Geometry check sheet. Reference: the model listing, model coordinates, mm. A direction names the side the tool comes from. Round coordinates to 2 decimals unless told otherwise and drop trailing zeros. Write each loop counter-clockwise with the first axis right and the second up, starting at its lowest first coordinate (ties: lowest second). Pieces come first, ordered by that corner, then holes. Notation, with made-up numbers: (74.25, 12) -> (111.25, 12) arc R18 cw to (111.25, 19) -> close; hole circle Ø3 at (61.5, -20). An arc over 180 degrees is marked (long way). Put each result on its own line as item: value. Start each with the question number.
from build123d import *

# Parameters (mm, degrees)
SKETCH041_W             = 20
SKETCH041_H             = 20
PAD030_DEPTH            = 50
PAD030_FACE1_W          = 20
PAD030_FACE1_H          = 50
PAD031_DEPTH            = 100
SKETCH043_W             = 20
SKETCH043_H             = 12
POCKET008_DEPTH         = 100
BODY003_PLACEMENT_ANGLE = 45


with BuildPart() as part:
    # Sketch041 → Pad030 (new body)
    with BuildSketch(Plane.XY):
        with Locations((-89.365005, -120.837763)):
            Rectangle(SKETCH041_W, SKETCH041_H)
    extrude(amount=PAD030_DEPTH)

    # Pad030 Face1 → Pad031 (add)
    with BuildSketch(Plane(origin=(-89.365005, -110.837763, 25), x_dir=(1, 0, 0), z_dir=(0, 1, 0))):
        Rectangle(PAD030_FACE1_W, PAD030_FACE1_H)
    extrude(amount=PAD031_DEPTH)

    # Sketch043 (on Face8 of Pad031) → Pocket008 (cut)
    with BuildSketch(Plane(origin=(0, -10.837763, 0), x_dir=(-1, 0, 0), z_dir=(0, 1, 0))):
        with Locations((89.365005, 6)):
            Rectangle(SKETCH043_W, SKETCH043_H)
    extrude(amount=-POCKET008_DEPTH, mode=Mode.SUBTRACT)


with BuildPart() as part_1:
    # Body003 placement: moved
    add(part.part.moved(Location((-94, -46, 10))).rotate(Axis((-94, -46, 10), (0, 0, -1)), BODY003_PLACEMENT_ANGLE))


solid = part_1.part
(1) Set-up check for faces 1 (the flat face through (-235.47, -61.28, 16.08)), 2 (the flat face through (-249.806, -75.227, 34.65)): record each of +Z, -Z, +X, -X, +Y, -Y from which the full face is reachable in a straight line by a thin tool's end or side.
(2) Go/stop test with flat-tipped pins: pin 1 Ø12 at (y, z) = (6, 28.5) entering from -X; pin 2 Ø10 at (x, z) = (-224.5, 33) entering from -Y; pin 3 Ø6 at (y, z) = (-10, 54.5) entering from +X; pin 4 Ø12 at (x, y) = (-193.5, -44.5) entering from +Z. Record where each tip stops, or that it passes through.
(3) Sectioned sample at A-A (z = 48). Record the cut outline in (x, y).
(4) Material ranges on L1, parallel to Z at x = -177, y = -5.5; L2, parallel to X at y = -10.5, z = 56; L3, parallel to Y at x = -217, z = 41, recorded low to high. Write a range as from..to.
(5) Sectioned sample at B-B (x = -239.5). Record the cut outline in (y, z).
(6) Sectioned sample at C-C (y = -20.5). Record the cut outline in (x, z), and give its area (3 significant figures).
Found:
1. face 1: -Z, +X, +Y
1. face 2: +Z, -Z, -X, -Y
2. pin 1: x = -188.52
2. pin 2: y = -69.26
2. pin 3: x = -167.24
2. pin 4: through
3. outline: (-256.78, -68.25) -> (-242.64, -82.4) -> (-157.78, 2.46) -> (-171.93, 16.6) -> close
4. L1: 22..60
4. L2: -199.02..-170.74
4. L3: -56.76..-28.48
5. outline: (-79.26, 10) -> (-57.25, 10) -> (-57.25, 22) -> (-50.98, 22) -> (-50.98, 60) -> (-79.26, 60) -> close
6. outline: (-209.02, 22) -> (-180.74, 22) -> (-180.74, 60) -> (-209.02, 60) -> close
6. area: 1,070 mm2
